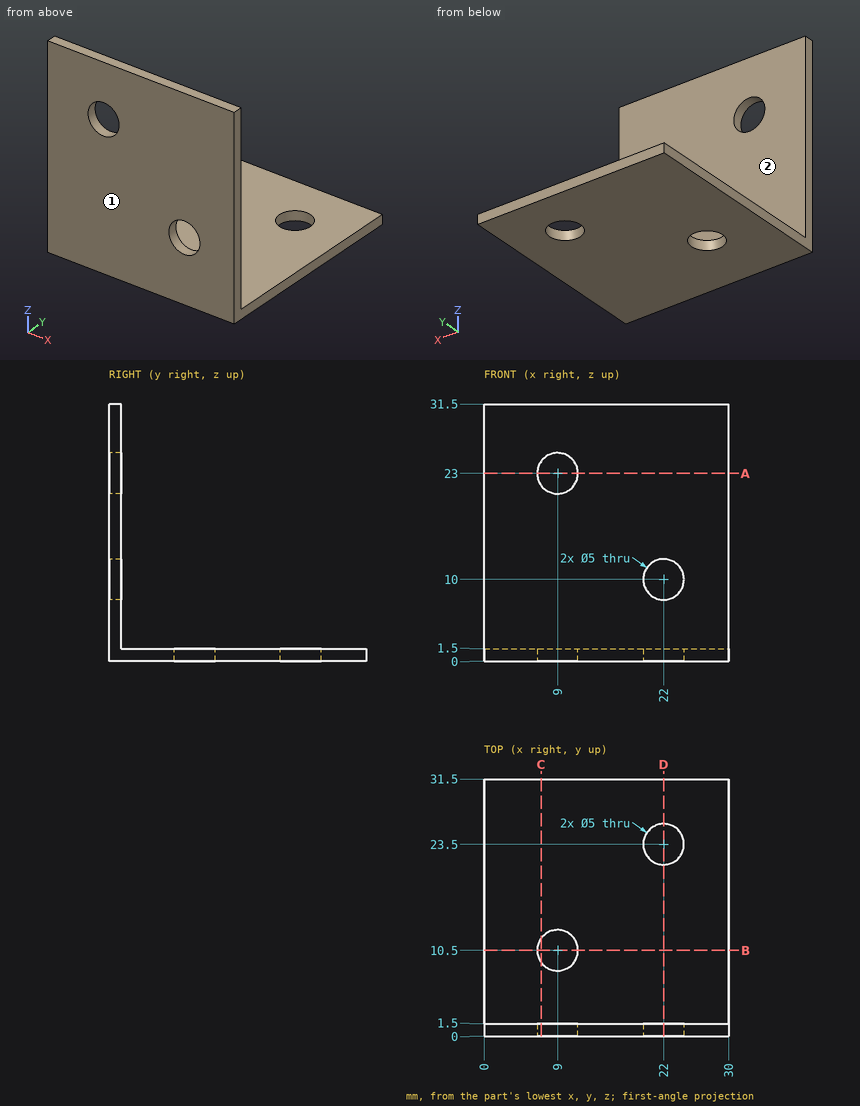
The figure shows three views and two pictorial views of one solid part (mm, origin at its lowest corner). Answer the questions. A direction names the side the tool comes from. Coordinates: 2 decimals unless noted, no trailing zeros. Write each loop counter-clockwise with the first axis right and the second up, starting at its lowest first coordinate (ties: lowest second). Pieces come first, ordered by that corner, then holes. Notation, with made-up numbers: (-29.75, -12.5) -> (3.25, -12.5) arc R13 cw to (3.25, -0.5) -> close; hole circle Ø1 at (78, 23). An arc over 180 degrees is marked (long way). Answer as a JSON object with one key per item and string values.
Q1. The part is cut by section A-A on z = 23. Give the vertices of the cut face in (x, y), then the cut area to 3 significant figures.
The answers:
{"outline": "(0, 0) -> (6.5, 0) -> (6.5, 1.5) -> (0, 1.5) -> close; (11.5, 0) -> (30, 0) -> (30, 1.5) -> (11.5, 1.5) -> close", "area": "37.5 mm2"}
Q2. A tool of negligible diameter and unlimited length cuts with its end or side. For the marked faces 1 and 2, from which of +Z, -Z, +X, -X, +Y, -Y can it reach the whole face along a straight path? Write none if from no direction.
The answers:
{"face 1": "+Z, -Z, +X, -X, -Y", "face 2": "+Z, +X, -X, +Y"}
Q3. The part is cut by section D-D on x = 22. Give the vertices of the cut face in (y, z).
The answers:
{"outline": "(0, 0) -> (21, 0) -> (21, 1.5) -> (1.5, 1.5) -> (1.5, 7.5) -> (0, 7.5) -> close; (0, 12.5) -> (1.5, 12.5) -> (1.5, 31.5) -> (0, 31.5) -> close; (26, 0) -> (31.5, 0) -> (31.5, 1.5) -> (26, 1.5) -> close"}
Q4. The part is cut by section C-C on x = 7. Give the vertices of the cut face in (y, z).
The answers:
{"outline": "(0, 0) -> (9, 0) -> (9, 1.5) -> (1.5, 1.5) -> (1.5, 21.5) -> (0, 21.5) -> close; (0, 24.5) -> (1.5, 24.5) -> (1.5, 31.5) -> (0, 31.5) -> close; (12, 0) -> (31.5, 0) -> (31.5, 1.5) -> (12, 1.5) -> close"}
Q5. Flat-ended cylindrical pins translate along their axes: pin 1 Ø3 at (x, z) = (8.5, 10.5) entering from +Y; pin 2 Ø9 at (x, y) = (21.5, 15) entering from +Z; pin 3 Ø3 at (x, z) = (9, 23) entering from +Y. Find the tip coordinate at first contact, or state that the pin passes through.
The answers:
{"pin 1": "stops at y = 1.5", "pin 2": "stops at z = 1.5", "pin 3": "passes through"}
Q6. Consider line 1 (Y direction, x = 9, z = 0.9); line 2 (X direction, y = 23.5, z = 0.85); line 3 (Y direction, x = 22, z = 1.05). Determine where each line is inside the solid, lowest interval first. Write a range as [from, to].
The answers:
{"line 1": "y = [0, 8], [13, 31.5]", "line 2": "x = [0, 19.5], [24.5, 30]", "line 3": "y = [0, 21], [26, 31.5]"}
